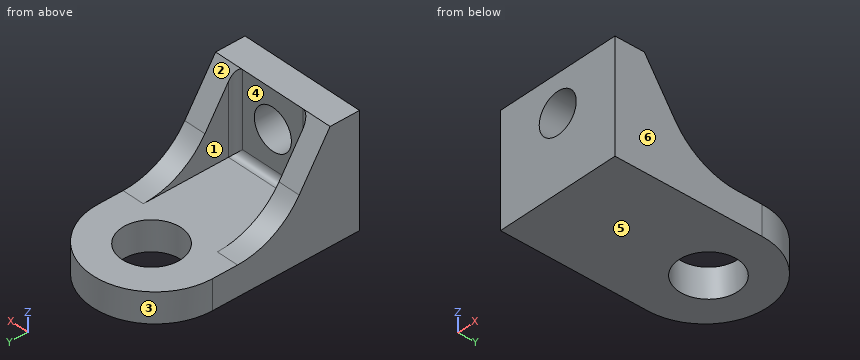
from build123d import *

# Parameters (mm, degrees)
RESSALTO_EXTRUS_O1_DEPTH = 15
CORTE_EXTRUS_O1_START    = -11
CORTE_EXTRUS_O1_DEPTH    = 11
CORTE_EXTRUS_O2_DEPTH    = 37.417715469
FILETE1_R                = 10
FILETE2_R                = 1
FURO_COM_FOLGA_DE_M51_D  = 5.5
ESBO_O7_R                = 4
CORTE_EXTRUS_O3_DEPTH    = 32.709619991


with BuildPart() as part:
    # Esboço1 → Ressalto-extrusão1 (new body)
    with BuildSketch(Plane.XY):
        with BuildLine():
            Line((-8.5, 0), (8.5, 0))
            Line((8.5, 0), (8.5, 20))
            ThreePointArc((8.5, 20), (0, 28.5), (-8.5, 20))
            Line((-8.5, 20), (-8.5, 0))
        make_face()
    extrude(amount=RESSALTO_EXTRUS_O1_DEPTH)

    # Esboço2 → Corte-extrusão1 (cut)
    with BuildSketch(Plane.XY.offset(15).offset(CORTE_EXTRUS_O1_START)):
        with BuildLine():
            Line((-5.5, 4), (5.5, 4))
            Line((5.5, 4), (5.5, 26.480740698))
            ThreePointArc((5.5, 26.480740698), (0, 28.5), (-5.5, 26.480740698))
            Line((-5.5, 26.480740698), (-5.5, 4))
        make_face()
    extrude(amount=CORTE_EXTRUS_O1_DEPTH, mode=Mode.SUBTRACT)

    # Esboço3 → Corte-extrusão2 (cut, through all)
    with BuildSketch(Plane(origin=(8.5, 0, 0), x_dir=(0, 0, -1), z_dir=(1, 0, 0))):
        Polygon((-15, 4), (-4, 11.163154524), (-4, 28.5), (-15, 28.5), align=None)
    extrude(amount=-CORTE_EXTRUS_O2_DEPTH, mode=Mode.SUBTRACT)

    # Filete1
    filete1_edges = [part.edges().sort_by_distance(p)[0] for p in [
        (-7, 11.163154524, 4),
        (7, 11.163154524, 4),
    ]]
    fillet(filete1_edges, radius=FILETE1_R)

    # Filete2
    filete2_edges = [part.edges().sort_by_distance(p)[0] for p in [
        (-5.5, 4, 9.5),
        (0, 4, 4),
        (5.5, 4, 9.5),
    ]]
    fillet(filete2_edges, radius=FILETE2_R)

    # Furo com folga de M51 (through all)
    with Locations(Plane(origin=(0, 4, 0), x_dir=(1, 0, 0), z_dir=(0, 1, 0))):
        with Locations((0, -10)):
            Hole(FURO_COM_FOLGA_DE_M51_D / 2)

    # Esboço7 → Corte-extrusão3 (cut, through all)
    with BuildSketch(Plane.XY.offset(4)):
        with Locations((0, 20.5)):
            Circle(ESBO_O7_R)
    extrude(amount=-CORTE_EXTRUS_O3_DEPTH, mode=Mode.SUBTRACT)


solid = part.part
Geometry check sheet. Reference: the model listing, model coordinates, mm. Face numbers are marked on the shaded views. A direction names the side the tool comes from. Round coordinates to 2 decimals unless told otherwise and drop trailing zeros. Order: outer loops, then holes, each group sorted by start corner. A loop starts at its lowest first (then second) coordinate and runs counter-clockwise, first axis right, second up. Notation, with made-up numbers: M -30.75,-18 L -19.75,-18 A16 cw -19.75,-3 Z; hole C -15.75,1.25 d4. An arc over 180 degrees is marked long. Write each question's results on one line, items separated by ' | '. Start each with the question number.
1. Cross-section at A-A on x = 0. Record the boundary of the cut face in (y, z), plus the area to 3 significant figures.
2. Cross-section at B-B on z = 10. Record the boundary of the cut face in (x, y), plus the area to 3 significant figures.
3. Set-up check for the marked faces 1 and 2: record each of +Z, -Z, +X, -X, +Y, -Y from which the full face is reachable in a straight line by a thin tool's end or side.
4. Cross-section at D-D on y = 3. Record the boundary of the cut face in (x, z), plus the area to 3 significant figures.
5. Cross-section at C-C on y = 21.5. Record the boundary of the cut face in (x, z).
6. Draft check along X on the marked faces 3, 4, 5 and 6. Enter one of: pulls with the +X half, pulls with the -X half, needs draft (parallel to the pull), parting line crosses it, or undercut.
7. Go/stop test with flat-tipped pins: P1, Ø5, axis at x = 6, y = 13.5, coming from the +Z side; P2, Ø8, axis at x = -1, z = 12, coming from the +Y side; P3, Ø1, axis at x = 5, y = 19.5, coming from the +Z side. Record where each tip stops, or that it passes through.
8. Material ranges on L1, parallel to Y at x = 0, z = 3.1; L2, parallel to X at y = 3.75, z = 10; L3, parallel to Z at x = 0, y = 1.6, recorded low to high. Write a range as from..to.
Resolved:
1) outline: M 0,0 L 16.5,0 L 16.5,4 L 5,4 A1 cw 4,5 L 4,7.25 L 0,7.25 Z; M 0,12.75 L 4,12.75 L 4,15 L 0,15 Z; M 24.5,0 L 28.5,0 L 28.5,4 L 24.5,4 Z | area: 104 mm2
2) outline: M -8.5,0 L -2.75,0 L -2.75,4 L -4.5,4 A1 cw -5.5,5 L -5.5,7.26 L -8.5,7.26 Z; M 2.75,0 L 8.5,0 L 8.5,7.26 L 5.5,7.26 L 5.5,5 A1 cw 4.5,4 L 2.75,4 Z | area: 66.0 mm2
3) face 1: +Z, +Y | face 2: +Z, +X, -X, +Y
4) outline: M -8.5,0 L 8.5,0 L 8.5,15 L -8.5,15 Z; hole C 0,10 d5.5 | area: 231 mm2
5) outline: M -8.37,0 L -3.87,0 L -3.87,4 L -8.37,4 Z; M 3.87,0 L 8.37,0 L 8.37,4 L 3.87,4 Z
6) face 3: parting line crosses it | face 4: undercut | face 5: needs draft | face 6: pulls with the +X half
7) P1: z = 5.7 | P2: y = 4.13 | P3: z = 4
8) L1: 0..16.5, 24.5..28.5 | L2: -8.5..-2.75, 2.75..8.5 | L3: 0..7.25, 12.75..15
